Could you check a few things on this drawing? It's one solid part, dimensions in mm from its lowest x, y, z. A direction names the side the tool comes from. Round coordinates to 2 decimals unless told otherwise and drop trailing zeros. Order: outer loops, then holes, each group sorted by start corner. A loop starts at its lowest first (then second) coordinate and runs counter-clockwise, first axis right, second up.
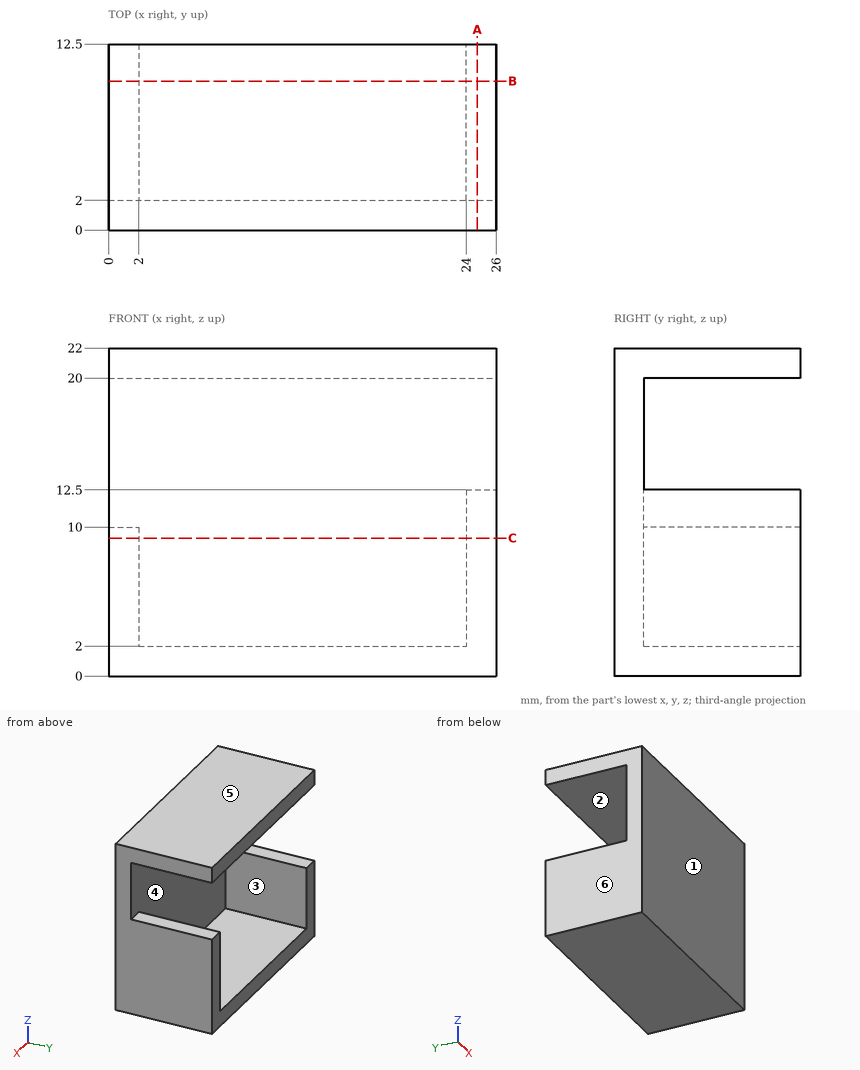
(1) I want a section at A-A, the plane x = 24.75. List the corners of the cut face in (y, z) for me.
(2) If we mould it in two halves opening along X, with no side actions, what happens to the marked faces 4, 5 and 6? For each: pulls with the +X half, pulls with the -X half, needs draft (parallel to the pull), parting line crosses it, or undercut.
(3) I'm going to push a flat-ended pin straight in: pin 1 Ø1.5 at (x, z) = (3, 3.5) entering from +Y. Where does the tip first touch, or does it pass through?
(4) Please list where these lines run through material, in increasing order: probe 1 along Z at (x, y) = (15, 8); probe 2 along X at (y, z) = (8.25, 3); probe 3 along Y at (x, z) = (12.25, 11.75).
(5) I want a section at C-C, the plane z = 9.25. List the corners of the cut face in (x, y) for me, plus the area to 3 significant figures.
(6) On a 3-axis mill with a long thin cutter (end or side, diameter ignored), from which of +Z, -Z, +X, -X, +Y, -Y can I reach the whole of each face in a straight line? I mean the marked faces 1, 2 and 3. Say none if no direction works.
(7) I want a section at B-B, the plane y = 10. List the corners of the cut face in (x, z) for me, plus the area to 3 significant figures.
Ans:
1. outline: (0, 0) - (12.5, 0) - (12.5, 12.5) - (2, 12.5) - (2, 20) - (12.5, 20) - (12.5, 22) - (0, 22) - close
2. face 4: undercut
2. face 5: needs draft
2. face 6: pulls with the -X half
3. pin 1: stops at y = 2
4. probe 1: z = 0 to 2, 20 to 22
4. probe 2: x = 0 to 2, 24 to 26
4. probe 3: y = 0 to 2
5. outline: (0, 0) - (26, 0) - (26, 12.5) - (24, 12.5) - (24, 2) - (2, 2) - (2, 12.5) - (0, 12.5) - close
5. area: 94.0 mm2
6. face 1: +Z, -Z, +X, -X, -Y
6. face 2: +X, -X, +Y
6. face 3: +Y
7. outline: (0, 0) - (26, 0) - (26, 12.5) - (24, 12.5) - (24, 2) - (2, 2) - (2, 10) - (0, 10) - close; (0, 20) - (26, 20) - (26, 22) - (0, 22) - close
7. area: 141 mm2
